The listing builds one solid part. Answer for the finished solid, in the listing's coordinates (mm). A direction names the side the tool comes from. Round coordinates to 2 decimals unless told otherwise and drop trailing zeros. Write each loop counter-clockwise with the first axis right and the second up, starting at its lowest first coordinate (ties: lowest second). Pieces come first, ordered by that corner, then holes. Notation, with made-up numbers: (-15.5, 8.25) - (37.5, 8.25) arc R17 cw to (37.5, 33.25) - close; hole circle Ø8 at (44, 41). An arc over 180 degrees is marked (long way). Return JSON: item names as keys, results as strings. Group by question number.
(1) Section C-C, the plane y = 2.5 is taken. Write down the section's boundary in (x, z), then the cut area to 3 significant figures.
(2) Which of the six approach directions +Z, -Z, +X, -X, +Y, -Y give full straight-line access (tool end or side, diameter ignored) to faces 1 (the cylindrical face through (22.394, 18.46, 15.26)), 2 (the flat face through (24, 11, 14.5)), 3 (the flat face through (0, 11, -14.5)), 4 (the flat face through (20, 11, 15)), 5 (the flat face through (0, 23, -15))?
(3) Section A-A, the plane x = 10 is taken. Write down the section's boundary in (y, z).
(4) Each of these flat-tipped pins is pushed along its axis until it touches: pin 1 (12 mm diameter, centred on x = 3.5, z = -6.5, fed in from +Y); pin 2 (1.5 mm diameter, centred on x = -1, y = 15, fed in from +Z); pin 3 (7 mm diameter, centred on x = 23.5, y = 6.5, fed in from -Z); pin 4 (4.5 mm diameter, centred on x = 20, z = 0, fed in from -Y). Where does it stop, or does it pass through?
(5) Section D-D, the plane x = 23.5 is taken. Write down the section's boundary in (y, z), then the cut area to 3 significant figures.
(6) Find the intervals of material crossed by line 1 along Y through (x, z) = (-23.5, 15.1); line 2 along X through (y, z) = (-0.5, 0); line 3 along Y through (x, z) = (23.5, 15.4), in increasing order. Write a range as [from, to].
(7) Section B-B, the plane z = 0 is taken. Write down the section's boundary in (x, y), then the cut area to 3 significant figures.
(8) Determine the mould class of faces 6 (the flat face through (-25, 11, 14.5)), 7 (the flat face through (18.5, 11, -15)), 8 (the cylindrical face through (-25, 8.26, 15.26)) for opening direction X: +X half, -X half, draft (parallel to the pull), parting line (faces both ways), or undercut.
```python
from build123d import *

# Parameters (mm, degrees)
SKETCH1_W           = 58
SKETCH1_H           = 32
BOSS_EXTRUDE1_DEPTH = 1.5
SKETCH1_3_W         = 9
SKETCH1_3_H         = 1.5
BOSS_EXTRUDE2_DEPTH = 23
SKETCH2_R           = 1.5
CUT_EXTRUDE1_DEPTH  = 49.928519291
SKETCH1_4_W         = 37
SKETCH1_4_H         = 1.5
BOSS_EXTRUDE3_DEPTH = 23
SKETCH3_R           = 2.5
CUT_EXTRUDE2_DEPTH  = 48.960921592
SKETCH1_5_R         = 2.5
CUT_EXTRUDE3_DEPTH  = 25


with BuildPart() as part:
    # Sketch1 → Boss-Extrude1 (new body)
    with BuildSketch(Plane(origin=(0, 0, 0), x_dir=(1, 0, 0), z_dir=(0, 1, 0))):
        Rectangle(SKETCH1_W, SKETCH1_H)
    extrude(amount=-BOSS_EXTRUDE1_DEPTH)

    # Sketch1_3 → Boss-Extrude2 (add)
    with BuildSketch(Plane(origin=(0, 0, 0), x_dir=(1, 0, 0), z_dir=(0, 1, 0))):
        with Locations((-24.5, -15.25)):
            Rectangle(SKETCH1_3_W, SKETCH1_3_H)
        with Locations((24.5, -15.25)):
            Rectangle(SKETCH1_3_W, SKETCH1_3_H)
    extrude(amount=BOSS_EXTRUDE2_DEPTH)

    # Sketch2 → Cut-Extrude1 (cut, through all)
    with BuildSketch(Plane.XY.offset(16)):
        with Locations((-23.5, 19.197487824)):
            Circle(SKETCH2_R)
        with Locations((-23.5, 8.197487824)):
            Circle(SKETCH2_R)
        with Locations((23.5, 17.446590768)):
            Circle(SKETCH2_R)
        with Locations((23.5, 8.197487824)):
            Circle(SKETCH2_R)
    extrude(amount=-CUT_EXTRUDE1_DEPTH, mode=Mode.SUBTRACT)

    # Sketch1_4 → Boss-Extrude3 (add)
    with BuildSketch(Plane(origin=(0, 0, 0), x_dir=(1, 0, 0), z_dir=(0, 1, 0))):
        with Locations((0, 15.25)):
            Rectangle(SKETCH1_4_W, SKETCH1_4_H)
    extrude(amount=BOSS_EXTRUDE3_DEPTH)

    # Sketch3 → Cut-Extrude2 (cut, through all)
    with BuildSketch(Plane.XY.offset(-14.5)):
        with Locations((10, 12.822039296)):
            Circle(SKETCH3_R)
    extrude(amount=-CUT_EXTRUDE2_DEPTH, mode=Mode.SUBTRACT)

    # Sketch1_5 → Cut-Extrude3 (cut)
    with BuildSketch(Plane(origin=(0, 0, 0), x_dir=(1, 0, 0), z_dir=(0, 1, 0))):
        with Locations(Location((20, 0, 0), (0, 0, 270))):
            Circle(SKETCH1_5_R)
        with Locations(Location((-20, 0, 0), (0, 0, 270))):
            Circle(SKETCH1_5_R)
    extrude(amount=-CUT_EXTRUDE3_DEPTH, mode=Mode.SUBTRACT)


solid = part.part
```
Working result:
{
 "1": {"outline": "(-29, 14.5) - (-20, 14.5) - (-20, 16) - (-29, 16) - close; (-18.5, -16) - (18.5, -16) - (18.5, -14.5) - (-18.5, -14.5) - close; (20, 14.5) - (29, 14.5) - (29, 16) - (20, 16) - close", "area": "82.5 mm^2"},
 "2": {"face 1": "+Z, -Z", "face 2": "-Z, +X, -X, +Y", "face 3": "+Z, +X, -X, +Y", "face 4": "+Z, -Z, +Y", "face 5": "+Z, -Z, +X, -X, +Y"},
 "3": {"outline": "(-1.5, -16) - (10.32, -16) - (10.32, -14.5) - (0, -14.5) - (0, 16) - (-1.5, 16) - close; (15.32, -16) - (23, -16) - (23, -14.5) - (15.32, -14.5) - close"},
 "4": {"pin 1": "stops at y = 0", "pin 2": "stops at z = -14.5", "pin 3": "stops at z = 14.5", "pin 4": "passes through"},
 "5": {"outline": "(-1.5, -16) - (0, -16) - (0, 14.5) - (6.7, 14.5) - (6.7, 16) - (-1.5, 16) - close; (9.7, 14.5) - (15.95, 14.5) - (15.95, 16) - (9.7, 16) - close; (18.95, 14.5) - (23, 14.5) - (23, 16) - (18.95, 16) - close", "area": "73.5 mm^2"},
 "6": {"line 1": "y = [-1.5, 6.7], [9.7, 17.7], [20.7, 23]", "line 2": "x = [-29, -22.5], [-17.5, 17.5], [22.5, 29]", "line 3": "y = [-1.5, 6.7], [9.7, 15.95], [18.95, 23]"},
 "7": {"outline": "(-29, -1.5) - (-22.5, -1.5) - (-22.5, 0) - (-29, 0) - close; (-17.5, -1.5) - (17.5, -1.5) - (17.5, 0) - (-17.5, 0) - close; (22.5, -1.5) - (29, -1.5) - (29, 0) - (22.5, 0) - close", "area": "72.0 mm^2"},
 "8": {"face 6": "draft", "face 7": "+X half", "face 8": "undercut"}
}
